Check sheet for the modelled part. Datum: model origin and axes. Units: mm. A direction names the side the tool comes from. Coordinates: 2 decimals unless noted, no trailing zeros. Loops run counter-clockwise (first coordinate to the right, second up) from the corner with the lowest first, then second, coordinate; pieces in that order, holes last. Notation, with made-up numbers: (60, 35.5) - (88, 35.5) arc R13 ccw to (88, 54.5) - close; hole circle Ø11 at (-18, -20.75). An arc over 180 degrees is marked (long way). Use a Markdown table: item, result. Add a question column.
1) Sectioned sample at A-A, the plane y = 0. Enter the section's corners in (x, z) (3 decimals), then the cut area to 3 significant figures.
2) Thickness scan on line 1 (Y direction, x = 0, z = 1.5); line 2 (Y direction, x = 0, z = -1.75); line 3 (X direction, y = 0.25, z = 3.25). Record the ranges inside material, lowest first.
3) Sectioned sample at C-C, the plane z = 2.75. Enter the section's corners in (x, y) (3 decimals), then the cut area to 3 significant figures.
4) Tool access check on faces 1 (the flat face through (-2, 3, 2.286)), 2 (the flat face through (3, -2, -4.826)), 3 (the flat face through (-1, 0, 8.255)). Record the directions out of +Z, -Z, +X, -X, +Y, -Y that give a thin tool (end or side, any length) a straight path to the whole face; none if there is none.
5) Go/stop test with flat-tipped pins: P1, Ø6, axis at y = -3, z = -3.5, coming from the -X side; P2, Ø2, axis at x = 3, z = -8.5, coming from the +Y side; P3, Ø1, axis at x = 5, z = 1.5, coming from the +Y side. Record where each tip stops, or that it passes through.
6) Sectioned sample at D-D, the plane y = 2. Enter the section's corners in (x, z) (3 decimals), then the cut area to 3 significant figures.
from build123d import *

# Parameters (mm, degrees)
SKETCH1_R           = 6.35
BOSS_EXTRUDE1_DEPTH = 2.286
SKETCH2_R           = 3.175
BOSS_EXTRUDE2_DEPTH = 8.255
SKETCH3_R           = 3.9878
BOSS_EXTRUDE3_DEPTH = 4.826
SKETCH4_R           = 3.175
BOSS_EXTRUDE4_DEPTH = 9.144
SKETCH5_R           = 0.362927277
CUT_EXTRUDE1_DEPTH  = 23.225


with BuildPart() as part:
    # Sketch1 → Boss-Extrude1 (new body)
    with BuildSketch(Plane.XY):
        Circle(SKETCH1_R)
    extrude(amount=BOSS_EXTRUDE1_DEPTH)

    # Sketch2 → Boss-Extrude2 (add)
    with BuildSketch(Plane(origin=(0, 0, 0), x_dir=(-1, 0, 0), z_dir=(0, 0, -1))):
        Circle(SKETCH2_R)
    extrude(amount=-BOSS_EXTRUDE2_DEPTH)

    # Sketch3 → Boss-Extrude3 (add)
    with BuildSketch(Plane(origin=(0, 0, 0), x_dir=(-1, 0, 0), z_dir=(0, 0, -1))):
        Circle(SKETCH3_R)
    extrude(amount=BOSS_EXTRUDE3_DEPTH)

    # Sketch4 → Boss-Extrude4 (add)
    with BuildSketch(Plane(origin=(0, 0, -4.826), x_dir=(-1, 0, 0), z_dir=(0, 0, -1))):
        Circle(SKETCH4_R)
    extrude(amount=BOSS_EXTRUDE4_DEPTH)

    # Sketch5 → Cut-Extrude1 (cut, through all)
    with BuildSketch(Plane.XY.offset(8.255)):
        Circle(SKETCH5_R)
    extrude(amount=-CUT_EXTRUDE1_DEPTH, mode=Mode.SUBTRACT)


solid = part.part
Solved:
| question | item | result |
|---|---|---|
| 1 | outline | (-6.35, 0) - (-3.988, 0) - (-3.988, -4.826) - (-3.175, -4.826) - (-3.175, -13.97) - (-0.363, -13.97) - (-0.363, 8.255) - (-3.175, 8.255) - (-3.175, 2.286) - (-6.35, 2.286) - close; (0.363, -13.97) - (3.175, -13.97) - (3.175, -4.826) - (3.988, -4.826) - (3.988, 0) - (6.35, 0) - (6.35, 2.286) - (3.175, 2.286) - (3.175, 8.255) - (0.363, 8.255) - close |
| 1 | area | 147 mm2 |
| 2 | line 1 | y = -6.35 to -0.36, 0.36 to 6.35 |
| 2 | line 2 | y = -3.99 to -0.36, 0.36 to 3.99 |
| 2 | line 3 | x = -3.17 to -0.26, 0.26 to 3.17 |
| 3 | outline | circle Ø6.35 at (0, 0); hole circle Ø0.726 at (0, 0) |
| 3 | area | 31.3 mm2 |
| 4 | face 1 | +Z |
| 4 | face 2 | -Z |
| 4 | face 3 | +Z, +X, -X, +Y, -Y |
| 5 | P1 | stops at x = -3.99 |
| 5 | P2 | stops at y = 2.47 |
| 5 | P3 | stops at y = 4.48 |
| 6 | outline | (-6.027, 0) - (-3.45, 0) - (-3.45, -4.826) - (-2.466, -4.826) - (-2.466, -13.97) - (2.466, -13.97) - (2.466, -4.826) - (3.45, -4.826) - (3.45, 0) - (6.027, 0) - (6.027, 2.286) - (2.466, 2.286) - (2.466, 8.255) - (-2.466, 8.255) - (-2.466, 2.286) - (-6.027, 2.286) - close |
| 6 | area | 135 mm2 |
